```python
from build123d import *

# Parameters (mm, degrees)
CROQUIS_PLANTA_R           = 7.5
SALIENTE_EXTRUIR1_DEPTH    = 20
SALIENTE_EXTRUIR2_DEPTH    = 45
SALIENTE_EXTRUIR3_DEPTH    = 75
CROQUIS14_R                = 6
CORTAR_EXTRUIR1_DEPTH      = 8.83956507
CORTAR_EXTRUIR1_DEPTH_BACK = 43.83956507


with BuildPart() as part:
    # Croquis Planta → Saliente-Extruir1 (new body)
    with BuildSketch(Plane(origin=(0, 0, 0), x_dir=(1, 0, 0), z_dir=(0, 1, 0))):
        with BuildLine():
            ThreePointArc((-6.856359495, -24.394341401), (-25.33956507, 0), (-6.856359495, 24.394341401))
            Line((-6.856359495, 24.394341401), (-75, 15))
            ThreePointArc((-75, 15), (-90, 0), (-75, -15))
            Line((-75, -15), (-6.856359495, -24.394341401))
        make_face()
        with Locations((-75, 0)):
            Circle(CROQUIS_PLANTA_R, mode=Mode.SUBTRACT)
        with BuildLine():
            ThreePointArc((75, -15), (90, 0), (75, 15))
            Line((75, 15), (6.856359495, 24.394341401))
            ThreePointArc((6.856359495, 24.394341401), (20.196914684, 15.302881924), (25.33956507, 0))
            ThreePointArc((25.33956507, 0), (20.196914684, -15.302881924), (6.856359495, -24.394341401))
            Line((6.856359495, -24.394341401), (75, -15))
        make_face()
        with Locations((75, 0)):
            Circle(CROQUIS_PLANTA_R, mode=Mode.SUBTRACT)
        with BuildLine():
            ThreePointArc((25.33956507, 0), (20.196914684, 15.302881924), (6.856359495, 24.394341401))
            Line((6.856359495, 24.394341401), (0, 25.33956507))
            Line((0, 25.33956507), (-6.856359495, 24.394341401))
            ThreePointArc((-6.856359495, 24.394341401), (-25.33956507, 0), (-6.856359495, -24.394341401))
            Line((-6.856359495, -24.394341401), (0, -25.33956507))
            Line((0, -25.33956507), (6.856359495, -24.394341401))
            ThreePointArc((6.856359495, -24.394341401), (20.196914684, -15.302881924), (25.33956507, 0))
        make_face()
    extrude(amount=SALIENTE_EXTRUIR1_DEPTH)

    # Croquis11 → Saliente-Extruir2 (add)
    with BuildSketch(Plane(origin=(0, 0, 0), x_dir=(1, 0, 0), z_dir=(0, 1, 0))):
        with BuildLine():
            ThreePointArc((24.204205377, 7.5), (21.845030009, 12.840880882), (18.326034976, 17.5))
            Line((18.326034976, 17.5), (-18.326034976, 17.5))
            ThreePointArc((-18.326034976, 17.5), (-21.845030009, 12.840880882), (-24.204205377, 7.5))
            Line((-24.204205377, 7.5), (24.204205377, 7.5))
        make_face()
        with BuildLine():
            ThreePointArc((18.326034976, 17.5), (13.05454839, 21.718018424), (6.856359495, 24.394341401))
            Line((6.856359495, 24.394341401), (0, 25.33956507))
            Line((0, 25.33956507), (-6.856359495, 24.394341401))
            ThreePointArc((-6.856359495, 24.394341401), (-13.05454839, 21.718018424), (-18.326034976, 17.5))
            Line((-18.326034976, 17.5), (18.326034976, 17.5))
        make_face()
        with BuildLine():
            Line((-18.326034976, -17.5), (18.326034976, -17.5))
            ThreePointArc((18.326034976, -17.5), (21.845030009, -12.840880882), (24.204205377, -7.5))
            Line((24.204205377, -7.5), (-24.204205377, -7.5))
            ThreePointArc((-24.204205377, -7.5), (-21.845030009, -12.840880882), (-18.326034976, -17.5))
        make_face()
        with BuildLine():
            Line((0, -25.33956507), (6.856359495, -24.394341401))
            ThreePointArc((6.856359495, -24.394341401), (13.05454839, -21.718018424), (18.326034976, -17.5))
            Line((18.326034976, -17.5), (-18.326034976, -17.5))
            ThreePointArc((-18.326034976, -17.5), (-13.05454839, -21.718018424), (-6.856359495, -24.394341401))
            Line((-6.856359495, -24.394341401), (0, -25.33956507))
        make_face()
    extrude(amount=SALIENTE_EXTRUIR2_DEPTH)

    # Croquis12 → Saliente-Extruir3 (add)
    with BuildSketch(Plane(origin=(0, 0, 0), x_dir=(1, 0, 0), z_dir=(0, 1, 0))):
        with BuildLine():
            ThreePointArc((24.204205377, 7.5), (21.845030009, 12.840880882), (18.326034976, 17.5))
            Line((18.326034976, 17.5), (-18.326034976, 17.5))
            ThreePointArc((-18.326034976, 17.5), (-21.845030009, 12.840880882), (-24.204205377, 7.5))
            Line((-24.204205377, 7.5), (24.204205377, 7.5))
        make_face()
        with BuildLine():
            Line((-18.326034976, -17.5), (18.326034976, -17.5))
            ThreePointArc((18.326034976, -17.5), (21.845030009, -12.840880882), (24.204205377, -7.5))
            Line((24.204205377, -7.5), (-24.204205377, -7.5))
            ThreePointArc((-24.204205377, -7.5), (-21.845030009, -12.840880882), (-18.326034976, -17.5))
        make_face()
    extrude(amount=SALIENTE_EXTRUIR3_DEPTH)

    # Croquis14 → Cortar-Extruir1 (cut, two sides)
    with BuildSketch(Plane(origin=(0, 0, -17.5), x_dir=(-1, 0, 0), z_dir=(0, 0, -1))) as cortar_extruir1_sk:
        with Locations((0, 60)):
            Circle(CROQUIS14_R)
    extrude(amount=CORTAR_EXTRUIR1_DEPTH, mode=Mode.SUBTRACT)
    extrude(cortar_extruir1_sk.sketch, amount=-CORTAR_EXTRUIR1_DEPTH_BACK, mode=Mode.SUBTRACT)


solid = part.part
```
Work out the finished part from the listing and answer in its coordinate system (mm). A direction names the side the tool comes from. Round coordinates to 2 decimals unless told otherwise and drop trailing zeros. Write each loop counter-clockwise with the first axis right and the second up, starting at its lowest first coordinate (ties: lowest second). Pieces come first, ordered by that corner, then holes. Notation, with made-up numbers: (27, -30) -> (66, -30) arc R27 cw to (66, -10) -> close; hole circle Ø3 at (82, 12). An arc over 180 degrees is marked (long way). Write each question's results on one line, items separated by ' | '.
Q1. Determine the mould class of faces 1 (the flat face through (0, 53, 17.5)), 2 (the cylindrical face through (4.42, 64.06, 12.43)), 3 (the flat face through (-1, 20, 0)), 4 (the cylindrical face through (90, 10, 0)) for opening direction Z: released by +Z, released by -Z, zero draft, split by the parting line, or undercut.
Data:
face 1: released by +Z | face 2: zero draft | face 3: undercut | face 4: split by the parting line
Q2. Which of the six approach directions +Z, -Z, +X, -X, +Y, -Y give full straight-line access (tool end or side, diameter ignored) to faces 5 (the flat face through (0, 75, 12)), 6 (the flat face through (0, 45, 20)), 7 (the flat face through (0, 47, 7.5)), 8 (the flat face through (0, 45, -21)), 9 (the cylindrical face through (-90, 10, 0))?
Data:
face 5: +Z, -Z, +X, -X, +Y | face 6: +Z, +X, -X, +Y | face 7: +X, -X, +Y | face 8: -Z, +X, -X, +Y | face 9: -X, +Y, -Y
Q3. Section B-B, the plane z = 0 is taken. Write down the section's boundary in (x, y).
Data:
outline: (-90, 0) -> (-82.5, 0) -> (-82.5, 20) -> (-90, 20) -> close; (-67.5, 0) -> (67.5, 0) -> (67.5, 20) -> (-67.5, 20) -> close; (82.5, 0) -> (90, 0) -> (90, 20) -> (82.5, 20) -> close
Q4. Straight lines are drawn through the part: line 1 along Y through (x, z) = (0, 15); line 2 along Z through (x, y) = (75, 15.25); line 3 along Z through (x, y) = (10, 60.5). For each, find the intervals that lie inside material, in ascending order. Write a range as [from, to].
Data:
line 1: [0, 54], [66, 75] | line 2: [-15, -7.5], [7.5, 15] | line 3: [-17.5, -7.5], [7.5, 17.5]
Q5. Section D-D, the plane z = 9.5 is taken. Write down the section's boundary in (x, y), then the cut area to 3 significant figures.
Data:
outline: (-86.61, 0) -> (86.61, 0) -> (86.61, 20) -> (23.49, 20) -> (23.49, 75) -> (-23.49, 75) -> (-23.49, 20) -> (-86.61, 20) -> close; hole circle Ø12 at (0, 60) | area: 5,940 mm^2
Q6. Flat-ended cylindrical pins translate along their axes: P1, Ø24, axis at x = -75, z = 0, coming from the +Y side; P2, Ø6.5, axis at x = -4, z = -23, coming from the +Y side; P3, Ø10, axis at x = 62.5, y = 22, coming from the +Z side (3 decimals); P4, Ø8, axis at x = 50.5, z = 17, coming from the -Y side. Find the tip coordinate at first contact, or state that the pin passes through.
Data:
P1: y = 20 | P2: y = 45 | P3: z = 17.355 | P4: y = 0
Q7. Section C-C, the plane y = 60 is taken. Write down the section's boundary in (x, z), then the cut area to 3 significant figures.
Data:
outline: (-24.2, -7.5) arc R25.34 ccw to (-18.33, -17.5) -> (-6, -17.5) -> (-6, -7.5) -> close; (-24.2, 7.5) -> (-6, 7.5) -> (-6, 17.5) -> (-18.33, 17.5) arc R25.34 ccw to start; (6, -17.5) -> (18.33, -17.5) arc R25.34 ccw to (24.2, -7.5) -> (6, -7.5) -> close; (6, 7.5) -> (24.2, 7.5) arc R25.34 ccw to (18.33, 17.5) -> (6, 17.5) -> close | area: 631 mm^2
Q8. Section A-A, the plane y = 41 is taken. Write down the section's boundary in (x, z), then the cut area to 3 significant figures.
Data:
outline: (-24.2, -7.5) arc R25.34 ccw to (-6.86, -24.39) -> (0, -25.34) -> (6.86, -24.39) arc R25.34 ccw to (24.2, -7.5) -> close; (-24.2, 7.5) -> (24.2, 7.5) arc R25.34 ccw to (6.86, 24.39) -> (0, 25.34) -> (-6.86, 24.39) arc R25.34 ccw to start | area: 1,260 mm^2
